Drawing for the job (mm, zero at the part's lowest x, y, z). A direction names the side the tool comes from. Round coordinates to 2 decimals unless told otherwise and drop trailing zeros. Loops run counter-clockwise (first coordinate to the right, second up) from the corner with the lowest first, then second, coordinate; pieces in that order, holes last. Notation, with made-up numbers: M 87.25,-18 L 137.25,-18 A22 ccw 137.25,-5 Z; hole C -15.75,-16 d11. An arc over 180 degrees is marked long. Answer in a Markdown table with one row per item.
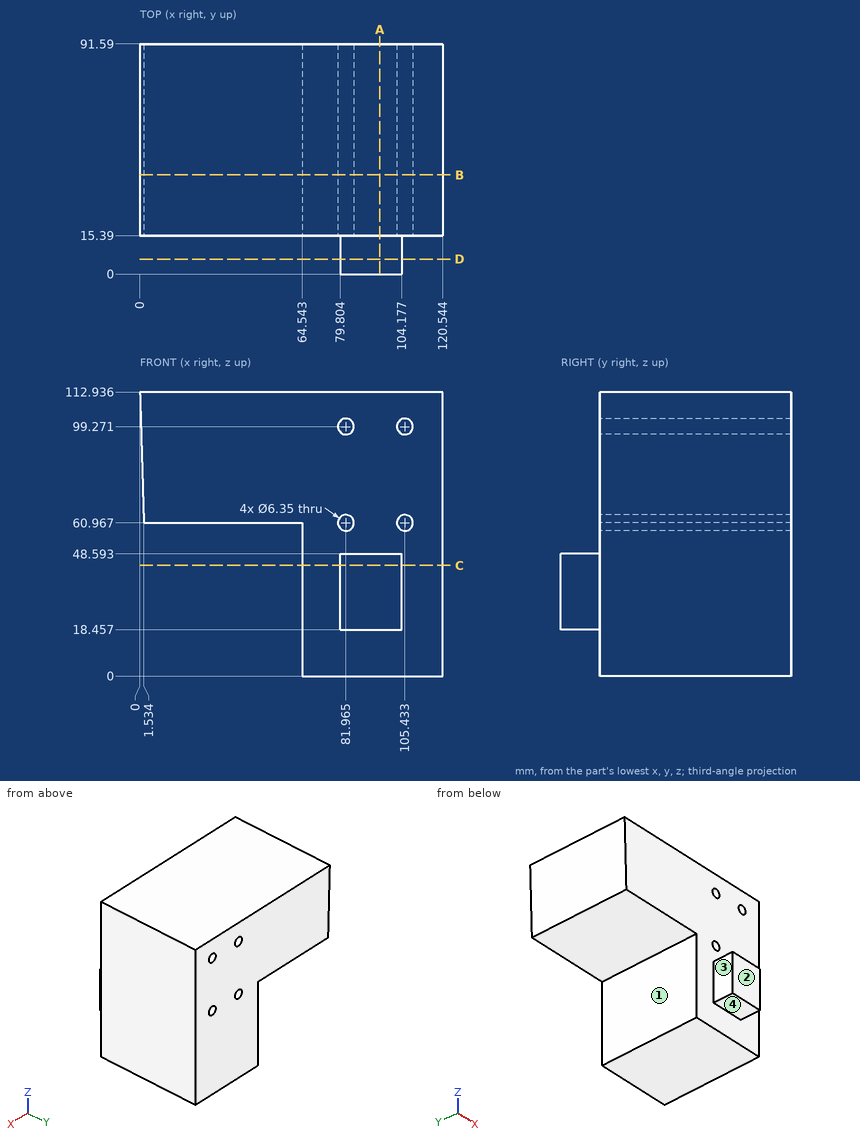
1. Pin check, flat tips, straight feed: pin 1 (8.5 mm diameter, centred on x = 81.96, z = 99.27, fed in from -Y); pin 2 (1.5 mm diameter, centred on x = 53, y = 43, fed in from -Z); pin 3 (4.5 mm diameter, centred on x = 89, y = 8.5, fed in from +Z); pin 4 (5.5 mm diameter, centred on x = 105.43, z = 99.27, fed in from -Y). Stop position of each tip, or through.
Verdict:
| item | result |
|---|---|
| pin 1 | stops at y = 15.39 |
| pin 2 | stops at z = 60.97 |
| pin 3 | stops at z = 48.59 |
| pin 4 | passes through |
2. Saw through at C-C (z = 44). Write the cut outline in (x, y) (1 decimal), and give its area (3 significant figures).
Verdict:
| item | result |
|---|---|
| outline | M 64.5,15.4 L 79.8,15.4 L 79.8,0 L 104.2,0 L 104.2,15.4 L 120.5,15.4 L 120.5,91.6 L 64.5,91.6 Z |
| area | 4,640 mm² |
3. Tool access for the marked faces 1, 2, 3 and 4: list every direction of +Z, -Z, +X, -X, +Y, -Y with a clear straight run to the whole face (end or side of a thin tool).
Verdict:
| item | result |
|---|---|
| face 1 | -Z, -X, +Y, -Y |
| face 2 | +Z, -Z, +X, -X, -Y |
| face 3 | +Z, -Z, -X, -Y |
| face 4 | -Z, +X, -X, -Y |
4. Saw through at D-D (y = 6). Write the cut outline in (x, z) (1 decimal).
Verdict:
| item | result |
|---|---|
| outline | M 79.8,18.5 L 104.2,18.5 L 104.2,48.6 L 79.8,48.6 Z |
5. Saw through at A-A (x = 95.5). Write the cut outline in (y, z) (1 decimal), and give its area (3 significant figures).
Verdict:
| item | result |
|---|---|
| outline | M 0,18.5 L 15.4,18.5 L 15.4,0 L 91.6,0 L 91.6,112.9 L 15.4,112.9 L 15.4,48.6 L 0,48.6 Z |
| area | 9,070 mm² |
6. Wall check: probe 1 along Z at (x, y) = (103, 84) (1 decimal); probe 2 along Z at (x, y) = (84.5, 77) (1 decimal); probe 3 along Z at (x, y) = (18.5, 75) (1 decimal). Give the ranges that are in metal, low to high.
Verdict:
| item | result |
|---|---|
| probe 1 | z = 0 to 58.9, 63 to 97.2, 101.3 to 112.9 |
| probe 2 | z = 0 to 59.1, 62.9 to 97.4, 101.2 to 112.9 |
| probe 3 | z = 61 to 112.9 |
7. Saw through at B-B (y = 39.5). State how many separate pieces and enclosed holes the cut face has, and give its area (3 significant figures).
Verdict:
| item | result |
|---|---|
| separate pieces | 1 |
| enclosed holes | 4 |
| area | 9,510 mm² |
